from build123d import *

# Parameters (mm, degrees)
SKETCH_1_R          = 10
EXTRUDE_1_DEPTH     = 2.5
SKETCH_2_R          = 4.5
EXTRUDE_2_DEPTH     = 3
SKETCH_3_R          = 3
CUT_EXTRUDE_1_DEPTH = 2.8
SKETCH_4_R          = 0.8
SKETCH_4_R_2        = 1.5
CUT_EXTRUDE_2_DEPTH = 16.173990905
CHAMFER_1_SIZE      = 0.3
SKETCH_5_R          = 4.5
SKETCH_5_R_2        = 3.5
SKETCH_5_R_3        = 3
SKETCH_5_R_4        = 1.5
CUT_EXTRUDE_3_DEPTH = 1


with BuildPart() as part:
    # 草图1 → 凸台-拉伸1 (new body)
    with BuildSketch(Plane(origin=(0, 0, 0), x_dir=(1, 0, 0), z_dir=(0, 1, 0))):
        with Locations(Location((0, 0, 0), (0, 0, 270))):
            Circle(SKETCH_1_R)
    extrude(amount=EXTRUDE_1_DEPTH)

    # 草图2 → 凸台-拉伸2 (add)
    with BuildSketch(Plane(origin=(0, 2.5, 0), x_dir=(1, 0, 0), z_dir=(0, 1, 0))):
        with Locations(Location((0, 0, 0), (0, 0, 270))):
            Circle(SKETCH_2_R)
    extrude(amount=EXTRUDE_2_DEPTH)

    # 草图3 → 切除-拉伸1 (cut)
    with BuildSketch(Plane(origin=(0, 5.5, 0), x_dir=(1, 0, 0), z_dir=(0, 1, 0))):
        with Locations(Location((0, 0, 0), (0, 0, 270))):
            Circle(SKETCH_3_R)
    extrude(amount=-CUT_EXTRUDE_1_DEPTH, mode=Mode.SUBTRACT)

    # 草图4 → 切除-拉伸2 (cut, through all)
    with BuildSketch(Plane.XZ):
        with Locations(Location((0, 7, 0), (0, 0, 270))):
            Circle(SKETCH_4_R)
        with Locations(Location((0, 0, 0), (0, 0, 270))):
            Circle(SKETCH_4_R_2)
        with Locations(Location((-3.25, 7, 0), (0, 0, 270))):
            Circle(SKETCH_4_R)
        with Locations(Location((3.25, 7, 0), (0, 0, 270))):
            Circle(SKETCH_4_R)
        with Locations(Location((7, 0, 0), (0, 0, 270))):
            Circle(SKETCH_4_R)
        with Locations(Location((7, 3.25, 0), (0, 0, 270))):
            Circle(SKETCH_4_R)
        with Locations(Location((7, -3.25, 0), (0, 0, 270))):
            Circle(SKETCH_4_R)
        with Locations(Location((0, -7, 0), (0, 0, 270))):
            Circle(SKETCH_4_R)
        with Locations(Location((3.25, -7, 0), (0, 0, 270))):
            Circle(SKETCH_4_R)
        with Locations(Location((-3.25, -7, 0), (0, 0, 270))):
            Circle(SKETCH_4_R)
        with Locations(Location((-7, 0, 0), (0, 0, 270))):
            Circle(SKETCH_4_R)
        with Locations(Location((-7, -3.25, 0), (0, 0, 270))):
            Circle(SKETCH_4_R)
        with Locations(Location((-7, 3.25, 0), (0, 0, 270))):
            Circle(SKETCH_4_R)
    extrude(amount=-CUT_EXTRUDE_2_DEPTH, mode=Mode.SUBTRACT)

    # 倒角1
    chamfer_1_edges = [part.edges().sort_by_distance(p)[0] for p in [
        (0, 5.5, -3),
        (0, 0, -10),
        (0, 2.5, -10),
        (0, 5.5, -4.5),
    ]]
    chamfer(chamfer_1_edges, length=CHAMFER_1_SIZE)

    # 草图5 → 切除-拉伸3 (cut)
    # profile 1 of 2: a face of its own
    with BuildSketch(Plane.XZ):
        with Locations(Location((0, 0, 0), (0, 0, 90))):
            Circle(SKETCH_5_R)
        with Locations(Location((0, 0, 0), (0, 0, 270))):
            Circle(SKETCH_5_R_2, mode=Mode.SUBTRACT)
    # profile 2 of 2: a face of its own
    with BuildSketch(Plane.XZ):
        with Locations(Location((0, 0, 0), (0, 0, 90))):
            Circle(SKETCH_5_R_3)
        with Locations(Location((0, 0, 0), (0, 0, 270))):
            Circle(SKETCH_5_R_4, mode=Mode.SUBTRACT)
    extrude(amount=-CUT_EXTRUDE_3_DEPTH, mode=Mode.SUBTRACT)


solid = part.part
Can you work these out from the model? Positions are in its coordinate system, mm. A direction names the side the tool comes from. Coordinates: 2 decimals unless noted, no trailing zeros. Answer as a JSON object with one key per item and string values. Group by question number.
Item 1: If we section it at A-A (x = 0): State how many separate pieces and enclosed holes the cut face has, plus the area to 3 significant figures.
Item 2: If I drill on L1, parallel to X at y = 0.55, z = 0; L2, parallel to X at y = 3.35, z = 0; L3, parallel to X at y = 1.6, z = -3.25, over which ranges is the centre line in solid material (lowest first)? Write a range as from..to.
Item 3: On a 3-axis mill with a long thin cutter (end or side, diameter ignored), from which of +Z, -Z, +X, -X, +Y, -Y can I reach the whole of each face in a straight line? I mean faces 4 (the face through (3.3, 1.2, -6.2)), 5 (the face through (-3.417, 0.493, 0.759)), 6 (the face through (-1.3, 2.7, 1.3)). Say none if no direction works.
Item 4: If we mould it in two halves opening along Z, with no side actions, what happens to faces 1 (the face through (-6.207, 1.232, -3.146)), 2 (the face through (-2, 5.5, -3)), 3 (the face through (1.352, 3.831, 4.292))? For each: released by +Z, released by -Z, zero draft, split by the parting line, or undercut.
Item 5: For pin 1 (2 mm diameter, centred on y = 5, z = 5, fed in from +X); pin 2 (2 mm diameter, centred on x = -7, z = 0, fed in from -Y); pin 3 (1.3 mm diameter, centred on x = -3.25, z = -7, fed in from -Y); pin 4 (1.8 mm diameter, centred on x = -7, z = 3.25, fed in from +Y), each with a flat end and sliding along its axis, tell me the tip position at first contact or that it passes through.
Returned:
{
 "1": {"separate pieces": "4", "enclosed holes": "0", "area": "38.7 mm²"},
 "2": {"L1": "x = -10..-7.8, -6.2..-4.5, -3.5..-3, 3..3.5, 4.5..6.2, 7.8..10", "L2": "x = -4.5..-3, 3..4.5", "L3": "x = -9.46..-7.8, -6.2..6.2, 7.8..9.46"},
 "3": {"face 4": "+Y, -Y", "face 5": "-Y", "face 6": "+Y"},
 "4": {"face 1": "undercut", "face 2": "zero draft", "face 3": "split by the parting line"},
 "5": {"pin 1": "stops at x = 2.06", "pin 2": "stops at y = 0", "pin 3": "passes through", "pin 4": "stops at y = 2.5"}
}
